For this review, take the finished solid that the model builds, in its own axes (mm). Face numbers are marked on the shaded views. A direction names the side the tool comes from. Give positions to 0.01 mm unless a question says otherwise; leave off trailing zeros. Write each loop counter-clockwise with the first axis right and the second up, starting at its lowest first coordinate (ties: lowest second). Pieces come first, ordered by that corner, then holes. Notation, with made-up numbers: M -13,-38.5 L 44,-38.5 A34 ccw 44,-6.5 Z; hole C -34.5,-18 d3. An arc over 180 degrees is marked long. One line per item, written item: value. Start each with the question number.
Item 1: Clearance check with flat-ended pins moving along their axes: pin 1 Ø4 at (y, z) = (-10.5, -6) entering from +X; pin 2 Ø6.5 at (x, y) = (5, -7.5) entering from -Z; pin 3 Ø5.5 at (x, y) = (14.5, 1.5) entering from +Z. State where each tip first meets the part, or that it passes through.
Item 2: Tool access review of the marked faces 1, 2, 3, 4 and 5: name each direction out of +Z, -Z, +X, -X, +Y, -Y from which nothing blocks a thin tool from reaching the whole face with its end or side.
Item 3: Consider section A-A, the plane y = -7. Write out the cut boundary in (x, z).
Item 4: To check wall thickness, follow probe 1 along Z at (x, y) = (1.35, -5); probe 2 along X at (y, z) = (-10.5, -7.75); probe 3 along Z at (x, y) = (4.75, -19). State the ranges of each line that lie inside material, in increasing order.
Item 5: Consider section D-D, the plane y = -15. Write out the cut boundary in (x, z).
Item 6: Consider section C-C, the plane x = 9. Write out the cut boundary in (y, z), and give its area (3 significant figures).
Autodesk Inventor part; units mm, degrees
ref_plane "Work Plane1" through (21, 0, 0) normal (1, 0, 0) x (0, 0, -1)
ref_plane "YZ Plane" through (0, 0, 0) normal (1, 0, 0) x (0, 1, 0)
ref_plane "XZ Plane" through (0, 0, 0) normal (0, 1, 0) x (-1, 0, 0)
sketch "Sketch1" plane through (0, 0, 0) normal (1, 0, 0) x (0, 1, 0)
  line L0 (0, 0) -> (5, 0)
  line L1 (5, 0) -> (5, -25)
  line L2 (5, -25) -> (0, -25)
  line L3 (0, -25) -> (0, 0)
  line L4 (0, 0) -> (-20, 0)
  line L5 (-20, 0) -> (-20, -20)
  line L6 (-20, -20) -> (0, -20)
  line L7 (0, -20) -> (0, 0)
  line L8 (-20, -10) -> (0, -10) construction
  circle A0 centre (-5, -10) radius 2.6
  circle A1 centre (-15, -10) radius 2.6
  dimension "d0" = 5
  dimension "d1" = 25
  dimension "d2" = 20
  dimension "d3" = 20
  dimension "d4" = 5.2
  dimension "d5" = 5.2
  dimension "d6" = 5
  dimension "d7" = 5
extrude "Extrusion1" add sketch "Sketch1" along normal blind 5
sketch "Sketch2" plane through (5, 0, 0) normal (1, 0, 0) x (0, 0, -1)
  line L0 (20, 0) -> (25, 0)
  line L1 (25, 5) -> (0, 5)
  line L2 (25, 0) -> (0, 0)
  line L3 (0, 0) -> (0, 5)
  line L4 (0, 5) -> (25, 5)
  line L5 (25, 5) -> (25, 0)
  line L6 (0, 0) -> (4, 0)
  line L7 (4, 0) -> (4, -8)
  line L8 (4, -8) -> (0, -8)
  line L9 (0, -8) -> (0, 0)
  line L10 (20, -20) -> (20, 0)
  line L11 (20, 0) -> (16, 0)
  line L12 (16, 0) -> (16, -8)
  line L13 (16, -8) -> (20, -8)
  line L14 (20, -8) -> (20, 0)
  line L15 (8.5, 0) -> (8.5, 5)
  point P0 (8.5, 5)
  dimension "d12" = 4
  dimension "d13" = 8
  dimension "d14" = 4
  dimension "d15" = 8
  dimension "d19" = 8.5
extrude "Extrusion2" add sketch "Sketch2" along normal blind 8 contours L2 L15 L1 L5 L0 | L10 L13 L12 L2
chamfer "Chamfer1" distance 8 angle 45 1 edges at (13, -8, -18)
sketch "Sketch3" plane through (13, 0, 0) normal (1, 0, 0) x (0, 0, -1)
  line L0 (8.5, 0) -> (8.5, 5)
  line L1 (16, 0) -> (8.5, 0)
  line L2 (8.5, 5) -> (8.5, 0)
  line L3 (8.5, 0) -> (11.5, 0)
  line L4 (11.5, 0) -> (11.5, 5)
  line L5 (25, 5) -> (0, 5)
  line L6 (11.5, 5) -> (8.5, 5)
  point P0 (0, 0)
  dimension "d20" = 3
ref_plane "Work Plane1" through (21, 0, 0) normal (1, 0, 0) x (0, 0, -1)
sketch "Sketch4" plane through (21, 0, 0) normal (1, 0, 0) x (0, 0, -1)
  line L0 (8.5, 0) -> (8.5, 5) construction
  line L1 (8.5, 2.5) -> (11.5, 2.5) construction
  line L2 (25, 5) -> (0, 5) construction
  line L3 (8.5, 2.7) -> (8.9, 2.7)
  line L4 (8.9, 2.7) -> (8.9, 2.3)
  line L5 (8.9, 2.3) -> (8.5, 2.3)
  line L6 (8.5, 2.3) -> (8.5, 2.7)
  point P0 (0, 0)
  dimension "d22" = 3
  dimension "d23" = 0.2
  dimension "d24" = 0.2
  dimension "d25" = 0.4
loft "Loft1" add profiles "Sketch3", "Sketch4"
equation "\"d7\" = d6"
equation "\"d24\" = d23"
properties part number "Z Axis Limt Adjustable Trigger"
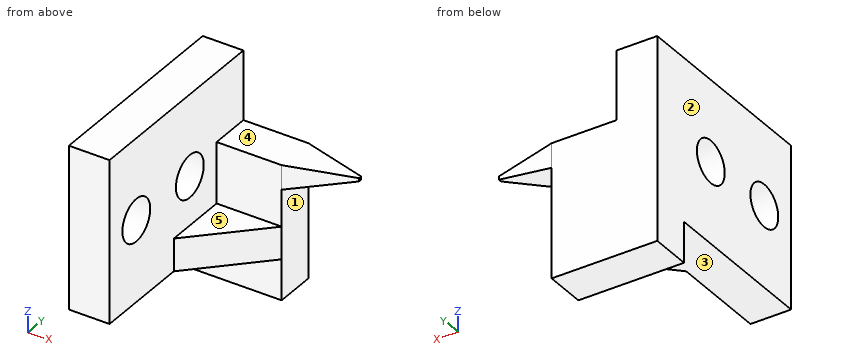
Model answer:
1. pin 1: stops at x = 5
1. pin 2: stops at z = -20
1. pin 3: stops at z = -8.5
2. face 1: -Z, +X, +Y, -Y
2. face 2: +Z, -Z, -X, +Y, -Y
2. face 3: -Z, +X, -X, -Y
2. face 4: +Z, +X, +Y, -Y
2. face 5: +Z, +X, -Y
3. outline: M 0,-20 L 6,-20 L 6,-16 L 5,-16 L 5,-11.66 L 0,-11.66 Z; M 0,-8.34 L 5,-8.34 L 5,0 L 0,0 Z
4. probe 1: z = -20 to -12.6, -7.4 to 0
4. probe 2: x = 0 to 5
4. probe 3: z = -20 to 0
5. outline: M 0,-20 L 5,-20 L 5,-12.6 L 0,-12.6 Z; M 0,-7.4 L 5,-7.4 L 5,0 L 0,0 Z
6. outline: M -4,-20 L 0,-20 L 0,-25 L 5,-25 L 5,-8.5 L 0,-8.5 L 0,-16 L -4,-16 Z
6. area: 98.5 mm2
